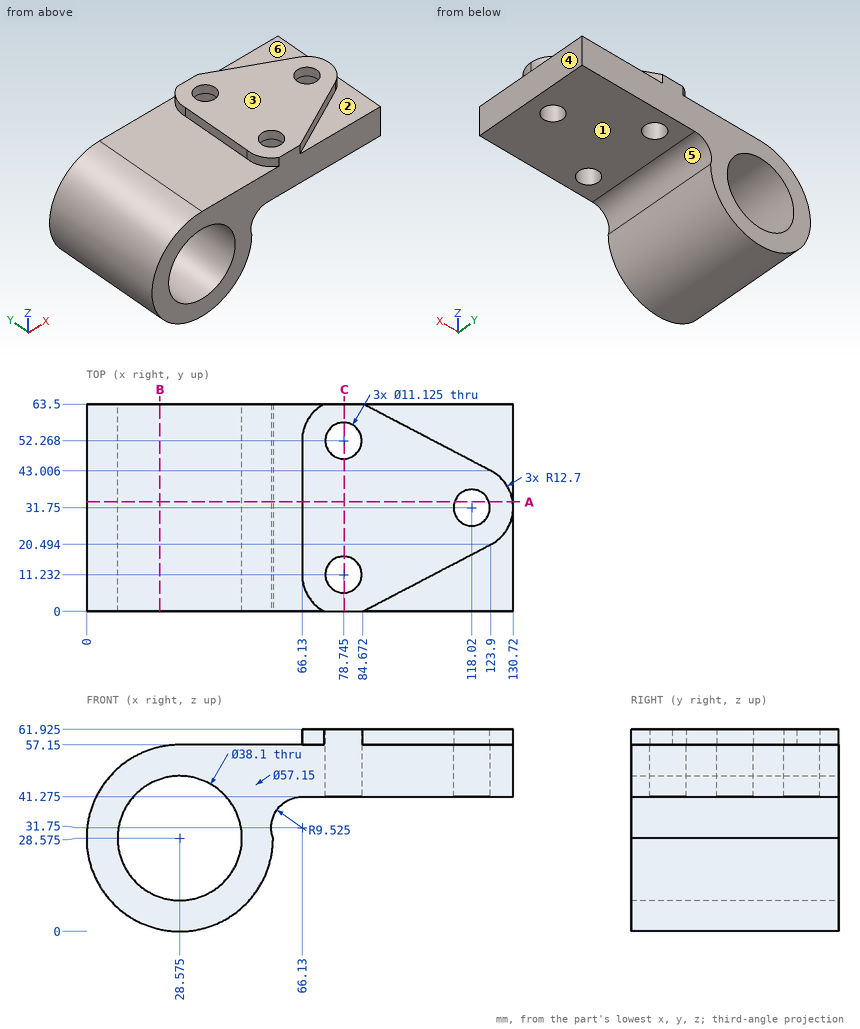
Print and shaded views of the part. All mm, measured from the part's lowest x, y and z. A direction names the side the tool comes from. Coordinates: 2 decimals unless noted, no trailing zeros. Write each loop counter-clockwise with the first axis right and the second up, starting at its lowest first coordinate (ties: lowest second). Pieces come first, ordered by that corner, then holes. Notation, with made-up numbers: M 28,3.5 L 59,3.5 A17 ccw 59,16.5 Z; hole C 20,89 d11. An arc over 180 degrees is marked long. Return JSON: item names as keys, results as strings.
1. Saw through at A-A, the plane y = 33.5. Count the separate pieces of the cut face and the enclosed holes in it, then the cut area to 3 significant figures.
Determined:
{"separate pieces": "2", "enclosed holes": "1", "area": "2,870 mm²"}
2. Flat gauge pins, fed straight in: pin 1 Ø14.5 at (x, y) = (118.02, 31.75) entering from -Z (1 decimal); pin 2 Ø2 at (x, y) = (61, 38.5) entering from +Z; pin 3 Ø5 at (y, z) = (33.5, 31.5) entering from +X. Where does each tip first touch, or does it go through?
Determined:
{"pin 1": "z = 41.3", "pin 2": "z = 57.15", "pin 3": "x = 57.01"}
3. Saw through at C-C, the plane x = 79. Write the cut outline in (y, z) (1 decimal).
Determined:
{"outline": "M 0,41.3 L 5.7,41.3 L 5.7,61.9 L 0,61.9 Z; M 16.8,41.3 L 46.7,41.3 L 46.7,61.9 L 16.8,61.9 Z; M 57.8,41.3 L 63.5,41.3 L 63.5,61.9 L 57.8,61.9 Z"}
4. Pull direction Z, two halves, no side cores. Call the marked faces 4, 5 and 6: pulls with the +Z half, pulls with the -Z half, needs draft (parallel to the pull), parting line crosses it, or undercut.
Determined:
{"face 4": "needs draft", "face 5": "undercut", "face 6": "pulls with the +Z half"}
5. 3-axis set-ups, long thin cutter, end or side, ignore diameter. For the marked faces 1, 2 and 3: which of +Z, -Z, +X, -X, +Y, -Y reach the whole face in a straight line?
Determined:
{"face 1": "-Z, +X, +Y, -Y", "face 2": "+Z, +X, -Y", "face 3": "+Z, +X, -X, +Y, -Y"}
6. Saw through at B-B, the plane x = 22.5. Write the cut outline in (y, z), then the cut area to 3 significant figures.
Determined:
{"outline": "M 0,0.65 L 63.5,0.65 L 63.5,10.52 L 0,10.52 Z; M 0,46.63 L 63.5,46.63 L 63.5,56.5 L 0,56.5 Z", "area": "1,250 mm²"}
7. Probe L1, parallel to Y at x = 82, z = 49 (1 decimal); L2, parallel to Z at x = 72, y = 56 (1 decimal); L3, parallel to X at y = 21, z = 45 (1 decimal). List the from-to ranges inside material, lowest first.
Determined:
{"L1": "0 to 6.7, 15.7 to 47.8, 56.8 to 63.5", "L2": "41.3 to 61.9", "L3": "5.2 to 18.9, 38.2 to 130.7"}
